Work out the finished part from the listing and answer in its coordinate system (mm). A direction names the side the tool comes from. Round coordinates to 2 decimals unless told otherwise and drop trailing zeros. Write each loop counter-clockwise with the first axis right and the second up, starting at its lowest first coordinate (ties: lowest second). Pieces come first, ordered by that corner, then holes.
from build123d import *

# Parameters (mm, degrees)
SKETCH1_W           = 13
SKETCH1_H           = 23
SKETCH1_W_2         = 3
SKETCH1_H_2         = 20
BOSS_EXTRUDE1_DEPTH = 3


with BuildPart() as part:
    # Sketch1 → Boss-Extrude1 (new body)
    with BuildSketch(Plane.XY):
        Polygon((-3, 70), (-3, 50), (0, 50), (0, 30), (-3, 30), (-3, 0), (0, 0), (62, 75.151515152), (62, 95), (59, 95), (59, 105), (15, 105), (-3, 105), (-3, 90), (0, 90), (0, 70), align=None)
        with Locations((45.5, 83.5)):
            Rectangle(SKETCH1_W, SKETCH1_H, mode=Mode.SUBTRACT)
        with Locations((30.5, 85)):
            Rectangle(SKETCH1_W_2, SKETCH1_H_2, mode=Mode.SUBTRACT)
    extrude(amount=BOSS_EXTRUDE1_DEPTH)


solid = part.part
Q1. Find section A-A (y = 81). Determine the outline of the cut face in (x, z).
Q2. Find section D-D (y = 64). Determine the outline of the cut face in (x, z).
Q3. Given pin 1 (0.9 mm diameter, centred on y = 81.5, z = 1, fed in from -X); pin 2 (1.5 mm diameter, centred on y = 101, z = 1.5, fed in from +X); pin 3 (10 mm diameter, centred on x = 53, y = 54, fed in from +Z); pin 4 (0.9 mm diameter, centred on x = 48.5, z = 2, fed in from -Y), each flat-ended and moving along its own axis, determine where each tip first touches the part or whether it passes through.
Q4. The mould has two halves that part along Y. Classify faces 1 (the face through (-1, 70, 1)), 2 (the face through (59, 100, 1)), 3 (the face through (28, 105, 1)): +Y half, -Y half, draft (parallel to the pull), parting line (faces both ways), or undercut.
Q5. A tool of negligible diameter and unlimited length cuts with its end or side. For faces 4 (the face through (32, 85, 1)), 5 (the face through (22, 65, 3)), 6 (the face through (-2, 90, 1)), from which of +Z, -Z, +X, -X, +Y, -Y can it reach the whole face along a straight path? Write none if from no direction.
Q6. Find section B-B (z = 2). Determine the outline of the cut face in (x, y).
Q7. Find the intervals of material crossed by L1, parallel to X at y = 78, z = 1.9; L2, parallel to Y at x = 31, z = 0.4; L3, parallel to X at y = 63, z = 1.45 (3 decimals), in increasing order.
Q8. Find section C-C (x = 16.5). Determine the outline of the cut face in (y, z).
Report:
1. outline: (0, 0) - (29, 0) - (29, 3) - (0, 3) - close; (32, 0) - (39, 0) - (39, 3) - (32, 3) - close; (52, 0) - (62, 0) - (62, 3) - (52, 3) - close
2. outline: (-3, 0) - (52.8, 0) - (52.8, 3) - (-3, 3) - close
3. pin 1: stops at x = 0
3. pin 2: stops at x = 59
3. pin 3: passes through
3. pin 4: stops at y = 58.24
4. face 1: undercut
4. face 2: draft
4. face 3: +Y half
5. face 4: +Z, -Z
5. face 5: +Z, +X, -X, +Y, -Y
5. face 6: +Z, -Z, -X
6. outline: (-3, 0) - (0, 0) - (62, 75.15) - (62, 95) - (59, 95) - (59, 105) - (-3, 105) - (-3, 90) - (0, 90) - (0, 70) - (-3, 70) - (-3, 50) - (0, 50) - (0, 30) - (-3, 30) - close; hole (29, 75) - (32, 75) - (32, 95) - (29, 95) - close; hole (39, 72) - (52, 72) - (52, 95) - (39, 95) - close
7. L1: x = 0 to 29, 32 to 39, 52 to 62
7. L2: y = 37.58 to 75, 95 to 105
7. L3: x = -3 to 51.975
8. outline: (20, 0) - (105, 0) - (105, 3) - (20, 3) - close
